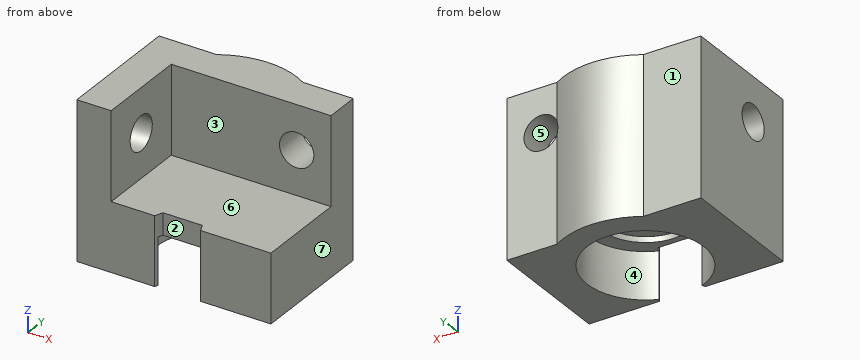
```python
from build123d import *

# Parameters (mm, degrees)
EXTRUDE_1_DEPTH     = 6
EXTRUDE_START       = 7.702227827
EXTRUDE_2_DEPTH     = 7.702227827
SKETCH_4_R          = 1.5
CUT_EXTRUDE_1_DEPTH = 6
SKETCH_5_R          = 1.5
CUT_EXTRUDE_2_DEPTH = 6


with BuildPart() as part:
    # Эскиз1 → Бобышка-Вытянуть1 (new body)
    with BuildSketch(Plane.XY):
        with BuildLine():
            Line((-416.117492961, 132.337705363), (-409.317492962, 132.337705363))
            Line((-409.317492962, 132.337705363), (-409.037492962, 133.037705363))
            Line((-409.037492962, 133.037705363), (-405.597492962, 133.037705363))
            Line((-405.597492962, 133.037705363), (-405.317492962, 132.337705363))
            Line((-405.317492962, 132.337705363), (-399.167492961, 132.337705363))
            Line((-399.167492961, 132.337705363), (-399.167492961, 143.47382058))
            Line((-399.167492961, 143.47382058), (-403.550784843, 143.47382058))
            ThreePointArc((-403.550784843, 143.47382058), (-407.317492962, 144.537705363), (-411.08420108, 143.47382058))
            Line((-411.08420108, 143.47382058), (-416.117492961, 143.47382058))
            Line((-416.117492961, 143.47382058), (-416.117492961, 132.337705363))
        make_face()
    extrude(amount=-EXTRUDE_1_DEPTH)

    # Эскиз2 → Вырез-Повернуть1 (revolve, cut)
    with BuildSketch(Plane(origin=(-407.317492962, 0, 0), x_dir=(0, 0, -1), z_dir=(1, 0, 0)), mode=Mode.PRIVATE) as cut_revolve_1_sk:
        Polygon((6.135092005, 142.437705363), (1.9, 142.437705363), (1.9, 141.109187411), (1.4, 141.109187411), (1.4, 137.337705363), (6.135092005, 137.337705363), align=None)
    revolve(cut_revolve_1_sk.sketch.rotate(Axis((-407.317492962, 137.337705363, -4.1), (0, 0, 1)), 90), axis=Axis((-407.317492962, 137.337705363, -4.1), (0, 0, 1)), mode=Mode.SUBTRACT)

    # Эскиз3 → Бобышка-Вытянуть2 (add)
    with BuildSketch(Plane.XY.offset(EXTRUDE_START)):
        with BuildLine():
            Line((-413.117492961, 140.47382058), (-413.117492961, 132.337705363))
            Line((-413.117492961, 132.337705363), (-416.117492961, 132.337705363))
            Line((-416.117492961, 132.337705363), (-416.117492961, 143.47382058))
            Line((-416.117492961, 143.47382058), (-411.08420108, 143.47382058))
            ThreePointArc((-411.08420108, 143.47382058), (-407.317492962, 144.537705363), (-403.550784843, 143.47382058))
            Line((-403.550784843, 143.47382058), (-399.167492961, 143.47382058))
            Line((-399.167492961, 143.47382058), (-399.167492961, 140.47382058))
            Line((-399.167492961, 140.47382058), (-413.117492961, 140.47382058))
        make_face()
    extrude(amount=-EXTRUDE_2_DEPTH)

    # Эскиз4 → Вырез-Вытянуть1 (cut)
    with BuildSketch(Plane(origin=(-413.117492961, 0, 0), x_dir=(0, 0, -1), z_dir=(1, 0, 0))):
        with Locations((-3.851113914, 136.405762972)):
            Circle(SKETCH_4_R)
    extrude(amount=-CUT_EXTRUDE_1_DEPTH, mode=Mode.SUBTRACT)

    # Эскиз5 → Вырез-Вытянуть2 (cut)
    with BuildSketch(Plane.XZ.offset(-140.47382058)):
        with Locations(Location((-402.167492961, 3.851113914, 0), (0, 0, 270))):
            Circle(SKETCH_5_R)
    extrude(amount=-CUT_EXTRUDE_2_DEPTH, mode=Mode.SUBTRACT)


solid = part.part
```
Input: part model. Units: mm. Frame: model coordinates. Face numbers are marked on the shaded views. A direction names the side the tool comes from. Give positions to 0.01 mm unless a question says otherwise; leave off trailing zeros. Order: outer loops, then holes, each group sorted by start corner. A loop starts at its lowest first (then second) coordinate and runs counter-clockwise, first axis right, second up. Notation, with made-up numbers: (52.25, -14.75) -> (70.25, -14.75) arc R33 ccw to (70.25, 18.25) -> close; hole circle Ø3 at (81.5, -22). An arc over 180 degrees is marked (long way). Write each question's results on one line, items separated by ' | '. Start each with the question number.
Item 1: Cut plane D-D on y = 138.25. Return the cut outline in (x, z).
Item 2: Cut plane C-C on z = 5. Return the cut outline in (x, y), then the cut area to 3 significant figures.
Item 3: Cut plane A-A on y = 135.25. Return the cut outline in (x, z), then the cut area to 3 significant figures.
Item 4: Contact query for flat-ended pins moving along their axis: P1, Ø4, axis at x = -405.5, z = -1, coming from the -Y side; P2, Ø6, axis at y = 135.5, z = 4.5, coming from the +X side; P3, Ø3.5, axis at x = -402.17, z = 3.85, coming from the +Y side; P4, Ø1, axis at x = -409, z = 5.5, coming from the -Y side. Output: stop coordinate, or through.
Item 5: Set-up query: the marked faces 1, 2, 3 and 4. Return all of +Z, -Z, +X, -X, +Y, -Y with unobstructed straight access to the full face (end or side cutting, diameter ignored); none if empty.
Item 6: Mould query, pull axis X, two halves, no side actions, for the marked faces 5, 6 and 7. Classes: pulls with the +X half, pulls with the -X half, needs draft (parallel to the pull), parting line crosses it, or undercut.
Item 7: Line query: line 1 (Y direction, x = -412, z = 2.75); line 2 (Y direction, x = -400.5, z = -0.25); line 3 (Z direction, x = -401, y = 137). Output: solid intervals per line, ascending.
Item 8: Cut plane B-B on x = -402.5. Return the cut outline in (y, z), then the cut area to 3 significant figures.
Established:
1) outline: (-416.12, -6) -> (-412.34, -6) -> (-412.34, -1.9) -> (-410.98, -1.9) -> (-410.98, -1.4) -> (-403.66, -1.4) -> (-403.66, -1.9) -> (-402.3, -1.9) -> (-402.3, -6) -> (-399.17, -6) -> (-399.17, 0) -> (-413.12, 0) -> (-413.12, 7.7) -> (-416.12, 7.7) -> close
2) outline: (-416.12, 132.34) -> (-413.12, 132.34) -> (-413.12, 135.44) -> (-416.12, 135.44) -> close; (-416.12, 137.37) -> (-413.12, 137.37) -> (-413.12, 140.47) -> (-403.13, 140.47) -> (-403.13, 143.47) -> (-403.55, 143.47) arc R7.2 ccw to (-411.08, 143.47) -> (-416.12, 143.47) -> close; (-401.2, 140.47) -> (-399.17, 140.47) -> (-399.17, 143.47) -> (-401.2, 143.47) -> close | area: 69.1 mm^2
3) outline: (-416.12, -6) -> (-411.97, -6) -> (-411.97, -1.9) -> (-410.46, -1.9) -> (-410.46, -1.4) -> (-404.18, -1.4) -> (-404.18, -1.9) -> (-402.66, -1.9) -> (-402.66, -6) -> (-399.17, -6) -> (-399.17, 0) -> (-413.12, 0) -> (-413.12, 2.89) -> (-416.12, 2.89) -> close; (-416.12, 4.81) -> (-413.12, 4.81) -> (-413.12, 7.7) -> (-416.12, 7.7) -> close | area: 77.8 mm^2
4) P1: y = 132.34 | P2: x = -413.12 | P3: y = 143.69 | P4: y = 140.47
5) face 1: +Z, -Z, -X, +Y | face 2: +Z, -Z, -Y | face 3: +Z, +X, -Y | face 4: -Z
6) face 5: undercut | face 6: needs draft | face 7: pulls with the +X half
7) line 1: 140.47 to 143.47 | line 2: 132.34 to 143.47 | line 3: -6 to 0
8) outline: (132.34, -6) -> (135.66, -6) -> (135.66, -1.9) -> (139.01, -1.9) -> (139.01, -6) -> (143.47, -6) -> (143.47, 2.39) -> (140.47, 2.39) -> (140.47, 0) -> (132.34, 0) -> close; (140.47, 5.31) -> (143.47, 5.31) -> (143.47, 7.7) -> (140.47, 7.7) -> close | area: 67.4 mm^2
